The figure shows three views and two pictorial views of one solid part (mm, origin at its lowest corner). Answer the questions. Coordinates: 2 decimals unless noted, no trailing zeros. Loops run counter-clockwise (first coordinate to the right, second up) from the corner with the lowest first, then second, coordinate; pieces in that order, holes last. Notation, with made-up numbers: M 74.5,69 L 106.5,69 A20 cw 106.5,93 Z; hole C 69.5,47 d10. An arc over 180 degrees is marked long. Answer as a JSON object with one key per item and string values. Group by question number.
1. A cutting plane is placed at A-A on x = 6.5. Give the vertices of the cut face in (y, z).
2. Determine the mould class of the marked faces 1, 2 and 3 for opening direction X: released by +X, released by -X, zero draft, split by the parting line, or undercut.
3. Given pin 1 (2 mm diameter, centred on x = 10.5, z = 1.5, fed in from -Y); pin 2 (2 mm diameter, centred on x = 9.5, z = 2.5, fed in from +Y) (1 decimal); pin 3 (1.5 mm diameter, centred on y = 5.5, z = 4, fed in from +X) (1 decimal), each flat-ended and moving along its own axis, determine where each tip first touches the part or whether it passes through.
4. Straight lines are drawn through the part: L1, parallel to Y at x = 6.5, z = 3.8; L2, parallel to Y at x = 5.25, z = 3.65; L3, parallel to X at y = 7, z = 3.55. For each, find the intervals that lie inside material, in ascending order.
5. A cutting plane is placed at C-C on z = 2.35. Give the vertices of the cut face in (x, y), and give its area (3 significant figures).
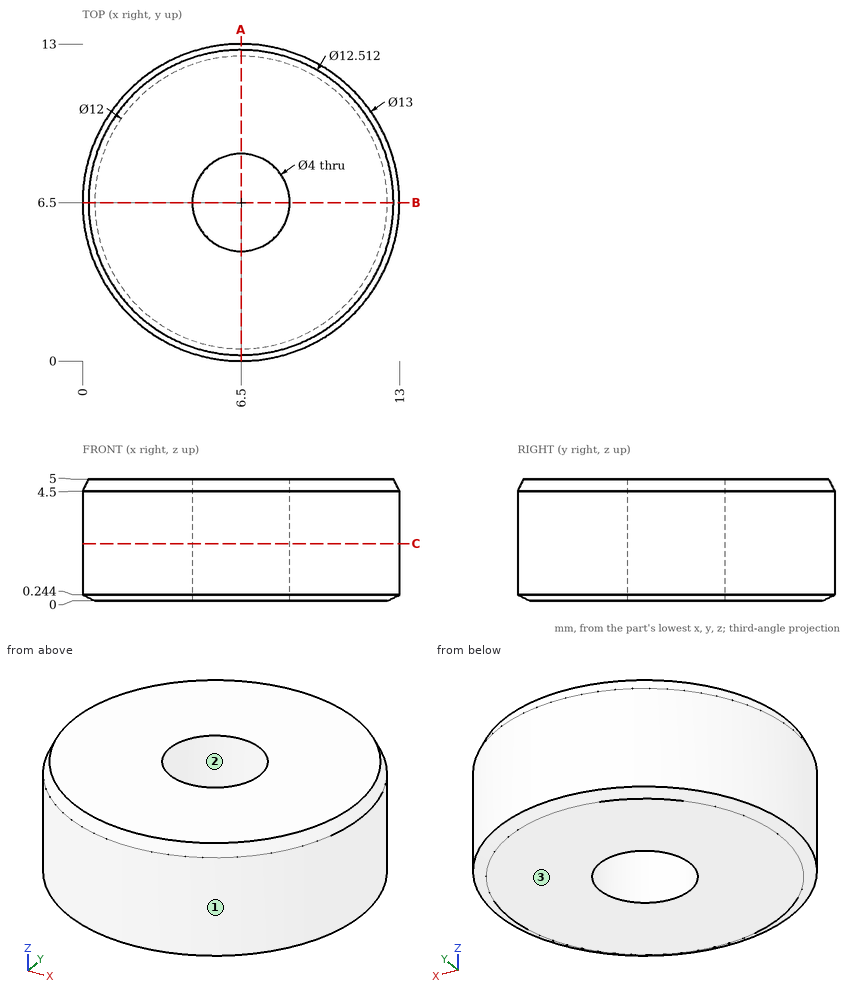
From the geometry:
{
 "1": {"outline": "M 0,0.24 L 0.5,0 L 4.5,0 L 4.5,5 L 0.24,5 L 0,4.5 Z; M 8.5,0 L 12.5,0 L 13,0.24 L 13,4.5 L 12.76,5 L 8.5,5 Z"},
 "2": {"face 1": "split by the parting line", "face 2": "undercut", "face 3": "zero draft"},
 "3": {"pin 1": "stops at y = 0.73", "pin 2": "stops at y = 12.7", "pin 3": "stops at x = 13"},
 "4": {"L1": "y = 0 to 4.5, 8.5 to 13", "L2": "y = 0.12 to 4.94, 8.06 to 12.88", "L3": "x = 0.02 to 4.56, 8.44 to 12.98"},
 "5": {"outline": "C 6.5,6.5 d13; hole C 6.5,6.5 d4", "area": "120 mm²"}
}
